The model under review builds one solid part; all positions refer to its coordinate system, in mm. Face numbers are marked on the shaded views. A direction names the side the tool comes from. Coordinates: 2 decimals unless noted, no trailing zeros. Loops run counter-clockwise (first coordinate to the right, second up) from the corner with the lowest first, then second, coordinate; pieces in that order, holes last. Notation, with made-up numbers: M 41,-3 L 80,-3 A13 cw 80,17 Z; hole C -27,-31.75 d7. An arc over 180 degrees is marked long. Use CSV: the item, a comma, the result in double quotes. Start each with the question number.
1. Tool access review of the marked faces 1 and 2: name each direction out of +Z, -Z, +X, -X, +Y, -Y from which nothing blocks a thin tool from reaching the whole face with its end or side.
2. Add section B-B, the plane x = 2.5. Write out the cut boundary in (y, z).
3. Clearance check with flat-ended pins moving along their axes: P1, Ø3, axis at x = 9, y = -1, coming from the -Z side; P2, Ø1.5, axis at x = 7, z = 0.5, coming from the +Y side; P3, Ø1.5, axis at y = 2.5, z = 0.5, coming from the +X side. State where each tip first meets the part, or that it passes through.
4. Add section A-A, the plane x = 13.75. Write out the cut boundary in (y, z).
5. Add section C-C, the plane y = 2.25. Write out the cut boundary in (x, z).
6. Draft analysis for pull direction Z (two halves, no side actions). For the marked faces 3, 4 and 5, state which applies: +Z half, -Z half, draft (parallel to the pull), parting line (faces both ways), or undercut.
7. For L1, parallel to Y at x = 11.75, z = 0; L2, parallel to X at y = -0.5, z = -3; L3, parallel to Y at x = 4.5, z = -1.75, list the stretches that pass through material, from the lowest coordinate up.
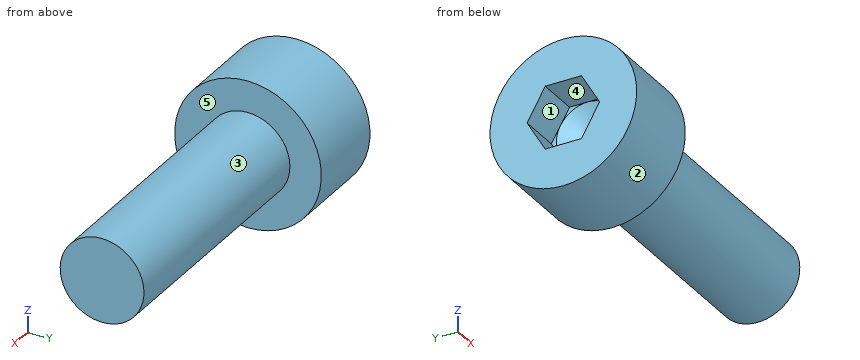
from build123d import *

# Parameters (mm, degrees)
CUT_EXTRUDE1_DEPTH = 2


with BuildPart() as part:
    # Sketch1 → Revolve1 (revolve)
    with BuildSketch(Plane.XY, mode=Mode.PRIVATE) as revolve1_sk:
        Polygon((0, 0), (0, 3.5), (4, 3.5), (4, 2), (16, 2), (16, 0), align=None)
    revolve(revolve1_sk.sketch.rotate(Axis((0, 0, 0), (1, 0, 0)), 90), axis=Axis((0, 0, 0), (1, 0, 0)))

    # Sketch2 → Cut-Revolve1 (revolve, cut)
    with BuildSketch(Plane.XY, mode=Mode.PRIVATE) as cut_revolve1_sk:
        Polygon((0, 1.5), (2, 1.5), (2.866025404, 0), (0, 0), align=None)
    revolve(cut_revolve1_sk.sketch.rotate(Axis((0, 0, 0), (1, 0, 0)), 180), axis=Axis((0, 0, 0), (1, 0, 0)), mode=Mode.SUBTRACT)

    # Sketch3 → Cut-Extrude1 (cut)
    with BuildSketch(Plane.ZY):
        Polygon((0, -1.732050808), (1.5, -0.866025404), (1.5, 0.866025404), (0, 1.732050808), (-1.5, 0.866025404), (-1.5, -0.866025404), align=None)
    extrude(amount=-CUT_EXTRUDE1_DEPTH, mode=Mode.SUBTRACT)


solid = part.part
Computed:
1,face 1,"-X"
1,face 2,"+X, -X"
2,outline,"C 0,0 d7; hole C 0,0 d1.27"
3,P1,"stops at z = -2"
3,P2,"stops at y = 2"
3,P3,"stops at x = 16"
4,outline,"C 0,0 d4"
5,outline,"M 0,-2.68 L 4,-2.68 L 4,2.68 L 0,2.68 Z"
6,face 3,"parting line"
6,face 4,"undercut"
6,face 5,"draft"
7,L1,"y = -2 to 2"
7,L2,"x = 0 to 4"
7,L3,"y = -0.97 to 0.97"
